Input: dimensioned drawing with shaded views. Units: mm. Origin: part minimum x, y, z. Give positions to 0.01 mm unless a question says otherwise; leave off trailing zeros. Write each loop counter-clockwise with the first axis right and the second up, starting at its lowest first coordinate (ties: lowest second). Pieces come first, ordered by that corner, then holes.
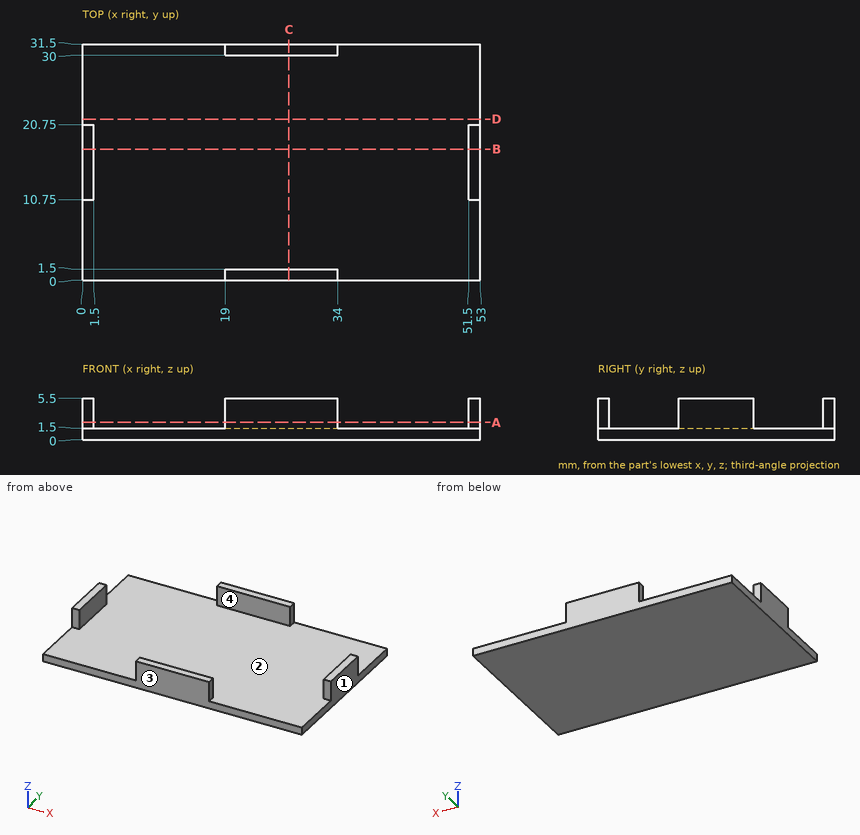
Item 1: Section B-B, the plane y = 17.5. Return the cut outline in (x, z), plus the area to 3 significant figures.
Found:
outline: (0, 0) - (53, 0) - (53, 5.5) - (51.5, 5.5) - (51.5, 1.5) - (1.5, 1.5) - (1.5, 5.5) - (0, 5.5) - close
area: 91.5 mm2
Item 2: Pull-direction query (Y, two-part tool) for the marked faces 1, 2, 3 and 4; classes: +Y half, -Y half, draft (parallel to the pull), parting line (faces both ways), or undercut.
Found:
face 1: draft
face 2: undercut
face 3: -Y half
face 4: undercut
Item 3: Section C-C, the plane x = 27.5. Return the cut outline in (y, z), plus the area to 4 significant figures.
Found:
outline: (0, 0) - (31.5, 0) - (31.5, 5.5) - (30, 5.5) - (30, 1.5) - (1.5, 1.5) - (1.5, 5.5) - (0, 5.5) - close
area: 59.25 mm2
Item 4: Section A-A, the plane z = 2.3. Return the cut outline in (x, y), plus the area to 3 significant figures.
Found:
outline: (0, 10.75) - (1.5, 10.75) - (1.5, 20.75) - (0, 20.75) - close; (19, 0) - (34, 0) - (34, 1.5) - (19, 1.5) - close; (19, 30) - (34, 30) - (34, 31.5) - (19, 31.5) - close; (51.5, 10.75) - (53, 10.75) - (53, 20.75) - (51.5, 20.75) - close
area: 75.0 mm2
Item 5: Section D-D, the plane y = 21.5. Return the cut outline in (x, z).
Found:
outline: (0, 0) - (53, 0) - (53, 1.5) - (0, 1.5) - close
Item 6: Pin query (flat end, axial travel): pin 1 Ø1.6 at (x, z) = (1, 3) entering from +Y; pin 2 Ø2 at (x, z) = (21, 2) entering from -Y; pin 3 Ø1.6 at (x, z) = (52, 3) entering from -Y; pin 4 Ø16 at (x, y) = (39.5, 11) entering from +Z. Return the tip coordinate at first contact, or that it passes through.
Found:
pin 1: stops at y = 20.75
pin 2: stops at y = 0
pin 3: stops at y = 10.75
pin 4: stops at z = 1.5
Item 7: Line query: L1, parallel to Y at x = 31.5, z = 1.95; L2, parallel to X at y = 17, z = 4.1; L3, parallel to Z at x = 28.5, y = 8. Output: solid intervals per line, ascending.
Found:
L1: y = 0 to 1.5, 30 to 31.5
L2: x = 0 to 1.5, 51.5 to 53
L3: z = 0 to 1.5
